Check sheet for the drawn part. Datum: minimum x, y, z corner. Units: mm. Give positions to 0.01 mm unless a question says otherwise; leave off trailing zeros. Order: outer loops, then holes, each group sorted by start corner. A loop starts at its lowest first (then second) coordinate and runs counter-clockwise, first axis right, second up.
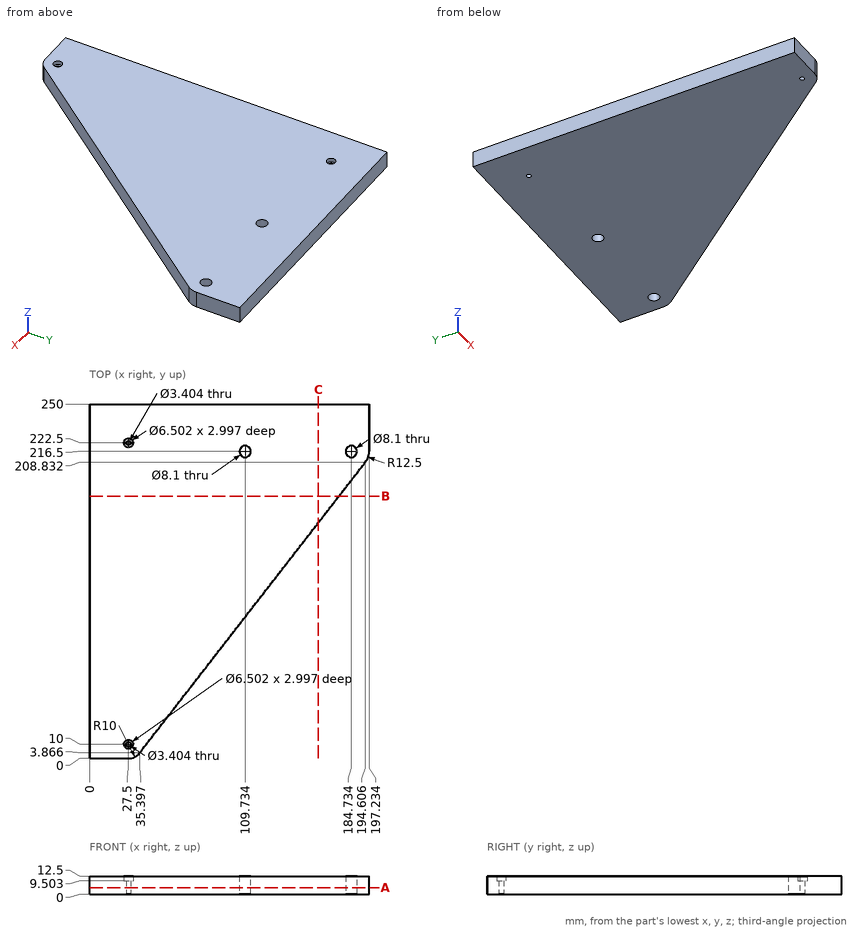
Item 1: Sectioned sample at C-C (x = 161.5). Enter the section's corners in (y, z), and give its area (3 significant figures).
Reported:
outline: (166.21, 0) - (250, 0) - (250, 12.5) - (166.21, 12.5) - close
area: 1,050 mm2
Item 2: Scan lines: L1, parallel to Y at x = 27.5, z = 11.9; L2, parallel to Y at x = 27.5, z = 4.5; L3, parallel to Y at x = 110, z = 5.75. Record each from-to range of solid material in increasing order.
Reported:
L1: y = 0 to 6.75, 13.25 to 219.25, 225.75 to 250
L2: y = 0 to 8.3, 11.7 to 220.8, 224.2 to 250
L3: y = 99.91 to 212.46, 220.54 to 250
Item 3: Sectioned sample at A-A (z = 4.5). Give the number of separate pieces and of enclosed holes in the cut face, and give its area (3 significant figures).
Reported:
separate pieces: 1
enclosed holes: 4
area: 31,700 mm2
Item 4: Gauge pin test, flat ends, axial feed: pin 1 (6.5 mm diameter, centred on x = 109.73, y = 216.5, fed in from +Z); pin 2 (1 mm diameter, centred on y = 171, z = 9, fed in from +X); pin 3 (5 mm diameter, centred on x = 27, y = 10, fed in from +Z). Record the tip position at first contact, or that the pin passes through.
Reported:
pin 1: passes through
pin 2: stops at x = 165.61
pin 3: stops at z = 9.5
Item 5: Sectioned sample at B-B (y = 185). Enter the section's corners in (x, z), and give its area (3 significant figures).
Reported:
outline: (0, 0) - (176.09, 0) - (176.09, 12.5) - (0, 12.5) - close
area: 2,200 mm2
